```python
from build123d import *

# Parameters (mm, degrees)
BOSS_EXTRUDE1_DEPTH = 2.5
SKETCH2_W           = 2
SKETCH2_H           = 47.5
BOSS_EXTRUDE2_DEPTH = 12
SKETCH3_W           = 5
SKETCH3_H           = 2
BOSS_EXTRUDE3_DEPTH = 5


with BuildPart() as part:
    # Sketch1 → Boss-Extrude1 (new body)
    with BuildSketch(Plane.XY):
        with BuildLine():
            Line((-20, 215), (-25, 215))
            Line((-25, 215), (-25, 225))
            Line((-25, 225), (-27, 225))
            Line((-27, 225), (-27, 213))
            Line((-27, 213), (-20, 213))
            Line((-20, 213), (-15.594125144, 198))
            Line((-15.594125144, 198), (-17.924730751, 188.7427864))
            ThreePointArc((-17.924730751, 188.7427864), (-18.746396058, 182.079894423), (-12.084524053, 181.25))
            Line((-12.084524053, 181.25), (12.084524053, 181.25))
            ThreePointArc((12.084524053, 181.25), (18.746396058, 182.079894423), (17.924730751, 188.7427864))
            Line((17.924730751, 188.7427864), (15.594125144, 198))
            Line((15.594125144, 198), (20, 213))
            Line((20, 213), (27, 213))
            Line((27, 213), (27, 225))
            Line((27, 225), (25, 225))
            Line((25, 225), (25, 215))
            Line((25, 215), (20, 215))
            Line((20, 215), (-20, 215))
        make_face()
        with BuildLine():
            ThreePointArc((-15, 181.25), (-17.957681098, 182.694653492), (-18.636522555, 185.915534655))
            ThreePointArc((-18.636522555, 185.915534655), (-14.538729788, 188.72152251), (-11.25, 185))
            ThreePointArc((-11.25, 185), (-12.348349571, 182.348349571), (-15, 181.25))
        make_face(mode=Mode.SUBTRACT)
        with BuildLine():
            ThreePointArc((18.75, 185), (17.651650429, 182.348349571), (15, 181.25))
            ThreePointArc((15, 181.25), (12.042318902, 187.305346508), (18.636522555, 185.915534655))
            ThreePointArc((18.636522555, 185.915534655), (18.72152251, 185.461270212), (18.75, 185))
        make_face(mode=Mode.SUBTRACT)
    extrude(amount=BOSS_EXTRUDE1_DEPTH)

    # Sketch2 → Boss-Extrude2 (add)
    with BuildSketch(Plane(origin=(0, 225, 0), x_dir=(1, 0, 0), z_dir=(0, 1, 0))):
        with Locations((26, -26.25)):
            Rectangle(SKETCH2_W, SKETCH2_H)
        with Locations((-26, -26.25)):
            Rectangle(SKETCH2_W, SKETCH2_H)
    extrude(amount=-BOSS_EXTRUDE2_DEPTH)

    # Sketch3 → Boss-Extrude3 (add)
    with BuildSketch(Plane.XY.offset(2.5)):
        with Locations((-22.5, 214)):
            Rectangle(SKETCH3_W, SKETCH3_H)
        with Locations((22.5, 214)):
            Rectangle(SKETCH3_W, SKETCH3_H)
    extrude(amount=BOSS_EXTRUDE3_DEPTH)


solid = part.part
```
Source: CAD feature listing. Evaluate the final solid. Frame: model axes, mm. A direction names the side the tool comes from. Give positions to 0.01 mm unless a question says otherwise; leave off trailing zeros. Loops run counter-clockwise (first coordinate to the right, second up) from the corner with the lowest first, then second, coordinate; pieces in that order, holes last. Notation, with made-up numbers: M 34,68.25 L 74,68.25 A9 cw 74,77.25 Z; hole C 30,-39.75 d2. An arc over 180 degrees is marked long. Put each result on its own line as item: value.
Q1. Pin query (flat end, axial travel): P1, Ø5.5, axis at x = -23.5, z = 16.5, coming from the -Y side; P2, Ø0.8, axis at x = -3.5, z = 2, coming from the -Y side; P3, Ø0.6, axis at x = 21.5, y = 213.5, coming from the +Z side. Return the tip coordinate at first contact, or that it passes through.
Response values:
P1: stops at y = 213
P2: stops at y = 181.25
P3: stops at z = 7.5
Q2. Reachability of faces 5 (the flat face through (16.776, 193.307, 1.232)), 6 (the flat face through (-16.743, 193.436, 1.232)), 7 (the flat face through (20, 214, 5)), 8 (the flat face through (0, 181.25, 1)), 9 (the flat face through (26, 213, 19)) from +Z, -Z, +X, -X, +Y, -Y: full face, straight path, thin tool, end or side. Return the list, or none.
Response values:
face 5: +Z, -Z, +X
face 6: +Z, -Z, -X
face 7: +Z, +Y, -Y
face 8: +Z, -Z, -Y
face 9: +Z, -Z, +X, -Y
Q3. Section B-B (z = 4). Return the cut outline in (x, y), and give its area (3 significant figures).
Response values:
outline: M -27,213 L -20,213 L -20,215 L -25,215 L -25,225 L -27,225 Z; M 20,213 L 27,213 L 27,225 L 25,225 L 25,215 L 20,215 Z
area: 68.0 mm²
Q4. Section D-D (y = 189.5). Return the cut outline in (x, z), and give its area (3 significant figures).
Response values:
outline: M -17.73,0 L 17.73,0 L 17.73,2.5 L -17.73,2.5 Z
area: 88.7 mm²
Q5. Line query: probe 1 along X at (y, z) = (185, 1); probe 2 along Y at (x, z) = (15, 1.75); probe 3 along X at (y, z) = (220, 14). Output: solid intervals per line, ascending. Write a range as [from, to].
Response values:
probe 1: x = [-19.75, -18.75], [-11.25, 11.25], [18.75, 19.75]
probe 2: y = [180.25, 181.25], [188.75, 215]
probe 3: x = [-27, -25], [25, 27]
Q6. Section A-A (z = 23). Return the cut outline in (x, y).
Response values:
outline: M -27,213 L -25,213 L -25,225 L -27,225 Z; M 25,213 L 27,213 L 27,225 L 25,225 Z
Q7. Mould query, pull axis Y, two halves, no side actions, for faces 1 (the flat face through (-26, 213, 19)), 2 (the flat face through (-17.828, 205.605, 1.232)), 3 (the flat face through (-23, 214, 7.5)), 4 (the flat face through (0, 215, 2)). Classes: released by +Y, released by -Y, zero draft, split by the parting line, or undercut.
Response values:
face 1: released by -Y
face 2: undercut
face 3: zero draft
face 4: released by +Y
Q8. Section C-C (x = -9). Return the cut outline in (y, z), and give its area (3 significant figures).
Response values:
outline: M 181.25,0 L 215,0 L 215,2.5 L 181.25,2.5 Z
area: 84.4 mm²
